Check sheet for the modelled part. Datum: model origin and axes. Units: mm. A direction names the side the tool comes from. Coordinates: 2 decimals unless noted, no trailing zeros. Loops run counter-clockwise (first coordinate to the right, second up) from the corner with the lowest first, then second, coordinate; pieces in that order, holes last. Notation, with made-up numbers: (-40, 10) - (17, 10) arc R31 ccw to (17, 49) - close; hole circle Ø4 at (-39, 63). An arc over 180 degrees is marked (long way). Write each question's results on one line, items separated by ' | '. Start each with the question number.
1. Cross-section at A-A (y = 4.3). Record the cut outline in (x, z).
2. Tool access check on faces 1 (the face through (15, 3, 20)), 2 (the face through (23, 3, 0)), 3 (the face through (7, 3, 0)). Record the directions out of +Z, -Z, +X, -X, +Y, -Y that give a thin tool (end or side, any length) a straight path to the whole face; none if there is none.
3. Cross-section at C-C (z = 12). Record the cut outline in (x, y).
4. Cross-section at B-B (x = 6.5). Record the cut outline in (y, z).
5. Thickness scan on line 1 (Z direction, x = 20.75, y = 0.9); line 2 (X direction, y = 3.6, z = 15). Record the ranges inside material, lowest first. Write a range as [from, to].
```python
from build123d import *

# Parameters (mm, degrees)
SKETCH1_W           = 3
SKETCH1_H           = 20
BOSS_EXTRUDE1_DEPTH = 5.08


with BuildPart() as part:
    # Sketch1 → Boss-Extrude1 (new body)
    with BuildSketch(Plane(origin=(0, 0, 0), x_dir=(1, 0, 0), z_dir=(0, 1, 0))):
        Polygon((13.5, 0), (16.5, 0), (30, 0), (30, 30), (0, 30), (0, 0), align=None)
        with Locations((15, -10)):
            Rectangle(SKETCH1_W, SKETCH1_H)
    extrude(amount=BOSS_EXTRUDE1_DEPTH)


solid = part.part
```
Established:
1) outline: (0, -30) - (30, -30) - (30, 0) - (16.5, 0) - (16.5, 20) - (13.5, 20) - (13.5, 0) - (0, 0) - close
2) face 1: +Z, +X, -X, +Y, -Y | face 2: +Z, +X, +Y, -Y | face 3: +Z, -X, +Y, -Y
3) outline: (13.5, 0) - (16.5, 0) - (16.5, 5.08) - (13.5, 5.08) - close
4) outline: (0, -30) - (5.08, -30) - (5.08, 0) - (0, 0) - close
5) line 1: [-30, 0] | line 2: [13.5, 16.5]
